```python
from build123d import *

# Parameters (mm, degrees)
F0_R     = 24.394867
F0_R_2   = 13.938556
F1_DEPTH = 25.4


with BuildPart() as f1:
    # F0 (on Front) → F1 (new body)
    with BuildSketch(Plane.XZ):
        with BuildLine():
            Line((9.7775, 37.878718), (0, 39.120286))
            ThreePointArc((0, 39.120286), (-39.120286, 0), (0, -39.120286))
            Line((0, -39.120286), (10.037051, -37.810771))
            ThreePointArc((10.037051, -37.810771), (31.008459, -23.851043), (39.120286, 0))
            ThreePointArc((39.120286, 0), (30.926488, 23.957235), (9.7775, 37.878718))
        make_face()
        Circle(F0_R, mode=Mode.SUBTRACT)
        with BuildLine():
            ThreePointArc((9.7775, 37.878718), (4.928007, 38.808653), (0, 39.120286))
            Line((0, 39.120286), (9.7775, 37.878718))
        make_face()
        with BuildLine():
            Line((10.037051, -37.810771), (0, -39.120286))
            ThreePointArc((0, -39.120286), (5.061058, -38.791526), (10.037051, -37.810771))
        make_face()
        with BuildLine():
            Line((136.504284, 21.786677), (9.7775, 37.878718))
            ThreePointArc((9.7775, 37.878718), (30.926488, 23.957235), (39.120286, 0))
            ThreePointArc((39.120286, 0), (31.008459, -23.851043), (10.037051, -37.810771))
            Line((10.037051, -37.810771), (134.907467, -21.519161))
            ThreePointArc((134.907467, -21.519161), (117.378733, 0.809535), (136.504284, 21.786677))
        make_face()
        with BuildLine():
            ThreePointArc((161.303011, 0), (153.833558, 16.504819), (136.504284, 21.786677))
            ThreePointArc((136.504284, 21.786677), (117.378733, 0.809535), (134.907467, -21.519161))
            ThreePointArc((134.907467, -21.519161), (153.215541, -17.027911), (161.303011, 0))
        make_face()
        with Locations((139.333412, 0)):
            Circle(F0_R_2, mode=Mode.SUBTRACT)
    extrude(amount=F1_DEPTH)


solid = f1.part
```
Work out the finished part from the listing and answer in its coordinate system (mm). Round coordinates to 2 decimals unless told otherwise and drop trailing zeros. Write each loop counter-clockwise with the first axis right and the second up, starting at its lowest first coordinate (ties: lowest second). Pieces come first, ordered by that corner, then holes. Notation, with made-up numbers: (-29.75, 0.5) - (21.25, 0.5) arc R17 ccw to (21.25, 13.5) - close; hole circle Ø11 at (26.25, 67.5). An arc over 180 degrees is marked (long way). Return JSON: item names as keys, results as strings. Group by question number.
Q1. The mould has two halves that part along X. Classify faces 1 (the cylindrical face through (5, -12.5, -38.8)), 2 (the flat face through (60, 0, 1)), 3 (the cylindrical face through (11.26, -12.52, -21.64)): released by +X, released by -X, zero draft, split by the parting line, or undercut.
Q2. The part is cut by section C-C on z = 6.5. Write down the section's boundary in (x, y), then the cut area to 3 significant figures.
Q3. The part is cut by section A-A on y = -7. Write down the section's boundary in (x, z), then the cut area to 3 significant figures.
Q4. The part is cut by section B-B on x = 22.5. Write down the section's boundary in (y, z), then the cut area to 3 significant figures.
Q5. Each of these flat-tipped pins is pushed along its axis until it touches: pin 1 Ø5 at (x, y) = (-4, -22.5) entering from -Z; pin 2 Ø1.5 at (x, y) = (3.5, -7.5) entering from -Z; pin 3 Ø4 at (x, y) = (-6, -21.5) entering from +Z. Where does it stop, or does it pass through?
Q6. Find the intervals of material crossed by L1, parallel to X at y = -6.75, z = 1; L2, parallel to X at y = -6, z = -7; L3, parallel to Z at x = -3, y = -12, in increasing order.
Q7. The part is cut by section D-D on x = 96. Write down the section's boundary in (y, z), then the cut area to 3 significant figures.
Solved:
{
 "1": {"face 1": "released by +X", "face 2": "zero draft", "face 3": "undercut"},
 "2": {"outline": "(-38.58, -25.4) - (-23.51, -25.4) - (-23.51, 0) - (-38.58, 0) - close; (23.51, -25.4) - (127, -25.4) - (127, 0) - (23.51, 0) - close; (151.66, -25.4) - (160.32, -25.4) - (160.32, 0) - (151.66, 0) - close", "area": "3,230 mm²"},
 "3": {"outline": "(0, -39.12) arc R39.12 ccw to (10.04, -37.81) - (134.91, -21.52) arc R21.97 ccw to (161.3, 0) arc R21.97 ccw to (136.5, 21.79) - (9.78, 37.88) arc R39.12 ccw to (0, 39.12) arc R39.12 ccw to start; hole circle Ø48.79 at (0, 0); hole circle Ø27.88 at (139.33, 0)", "area": "9,090 mm²"},
 "4": {"outline": "(-25.4, -36.18) - (0, -36.18) - (0, -9.43) - (-25.4, -9.43) - close; (-25.4, 9.43) - (0, 9.43) - (0, 36.26) - (-25.4, 36.26) - close", "area": "1,360 mm²"},
 "5": {"pin 1": "z = -39.09", "pin 2": "z = -39.02", "pin 3": "z = 38.92"},
 "6": {"L1": "-39.11 to -24.37, 24.37 to 125.43, 153.24 to 161.28", "L2": "-38.49 to -23.37, 23.37 to 127.28, 151.39 to 160.16", "L3": "-39.01 to -24.21, 24.21 to 39.01"},
 "7": {"outline": "(-25.4, -26.6) - (0, -26.6) - (0, 26.93) - (-25.4, 26.93) - close", "area": "1,360 mm²"}
}
